```python
from build123d import *

# Parameters (mm, degrees)
F0_W     = 177.8
F0_H     = 177.8
F1_DEPTH = 12.7
F2_D     = 6.8


# Not quite as in the source:
# - a length typed as a fraction of an inch, garbled in the dataset ("3 / 203.2 mm" for 3/8 in), is restored


with BuildPart() as f1:
    # F0 (on Front) → F1 (new body)
    with BuildSketch(Plane.XZ):
        with Locations((0, -7.6e-09)):
            Rectangle(F0_W, F0_H)
    extrude(amount=F1_DEPTH)

    # F2 (through all)
    with Locations(Plane(origin=(0, 0, 0), x_dir=(1, 0, 0), z_dir=(0, 1, 0))):
        with Locations((-61.9125, 7.6e-09), (0, -61.9124999924), (61.9125, 7.6e-09), (0, 61.9124999319)):
            Hole(F2_D / 2)


solid = f1.part
```
Check sheet for the modelled part. Datum: model origin and axes. Units: mm. Coordinates: 2 decimals unless noted, no trailing zeros. Write each loop counter-clockwise with the first axis right and the second up, starting at its lowest first coordinate (ties: lowest second). Pieces come first, ordered by that corner, then holes. Notation, with made-up numbers: (74.25, 3) -> (80.25, 3) arc R36 cw to (80.25, 42) -> close; hole circle Ø3 at (78, 74.25). An arc over 180 degrees is marked (long way). Use a Markdown table: item, result.
1. Sectioned sample at B-B (x = 0). Enter the section's corners in (y, z).
Reported:
| item | result |
|---|---|
| outline | (-12.7, -88.9) -> (0, -88.9) -> (0, -65.31) -> (-12.7, -65.31) -> close; (-12.7, -58.51) -> (0, -58.51) -> (0, 58.51) -> (-12.7, 58.51) -> close; (-12.7, 65.31) -> (0, 65.31) -> (0, 88.9) -> (-12.7, 88.9) -> close |
2. Scan lines: line 1 along Z through (x, y) = (0, -9.5); line 2 along Z through (x, y) = (-61, -3.5). Record each from-to range of solid material in increasing order.
Reported:
| item | result |
|---|---|
| line 1 | z = -88.9 to -65.31, -58.51 to 58.51, 65.31 to 88.9 |
| line 2 | z = -88.9 to -3.28, 3.28 to 88.9 |
3. Go/stop test with a flat-tipped pin: pin 1 Ø5.5 at (x, z) = (61.91, 0) entering from -Y. Record where the tip stops, or that it passes through.
Reported:
| item | result |
|---|---|
| pin 1 | passes through |
4. Release check for a two-part mould opening along Z. For faces 1 (the flat face through (-1, -6, -88.9)), 2 (the cylindrical face through (65.31, -6.44, -0.15)), 3 (the flat face through (88.9, -6, -1)) record: pulls with the +Z half, pulls with the -Z half, needs draft (parallel to the pull), parting line crosses it, or undercut.
Reported:
| item | result |
|---|---|
| face 1 | pulls with the -Z half |
| face 2 | undercut |
| face 3 | needs draft |
5. Sectioned sample at A-A (z = 0). Enter the section's corners in (x, y), plus the area to 3 significant figures.
Reported:
| item | result |
|---|---|
| outline | (-88.9, -12.7) -> (-65.31, -12.7) -> (-65.31, 0) -> (-88.9, 0) -> close; (-58.51, -12.7) -> (58.51, -12.7) -> (58.51, 0) -> (-58.51, 0) -> close; (65.31, -12.7) -> (88.9, -12.7) -> (88.9, 0) -> (65.31, 0) -> close |
| area | 2,090 mm2 |
